CAD build for the part. Positions are in the model's coordinates, mm. A direction names the side the tool comes from. Give positions to 0.01 mm unless a question says otherwise; leave off trailing zeros. Loops run counter-clockwise (first coordinate to the right, second up) from the corner with the lowest first, then second, coordinate; pieces in that order, holes last.
```python
from build123d import *

# Parameters (mm, degrees)
BOSS_EXTRUDE1_DEPTH = 5.35
SKETCH2_R           = 5
BOSS_EXTRUDE2_DEPTH = 1
SKETCH3_R           = 3.555
BOSS_EXTRUDE3_DEPTH = 2.5
SKETCH4_R           = 2.5
CUT_EXTRUDE1_DEPTH  = 9.85
CUT_EXTRUDE2_DEPTH  = 4.5


with BuildPart() as part:
    # Sketch1 → Boss-Extrude1 (new body)
    with BuildSketch(Plane(origin=(0, 0, 0), x_dir=(1, 0, 0), z_dir=(0, 1, 0))):
        Polygon((4.543746619, 0), (2.271873309, 3.935), (-2.271873309, 3.935), (-4.543746619, 0), (-2.271873309, -3.935), (2.271873309, -3.935), align=None)
    extrude(amount=BOSS_EXTRUDE1_DEPTH)

    # Sketch2 → Boss-Extrude2 (add)
    with BuildSketch(Plane(origin=(0, 0, 0), x_dir=(1, 0, 0), z_dir=(0, 1, 0))):
        Circle(SKETCH2_R)
    extrude(amount=-BOSS_EXTRUDE2_DEPTH)

    # Sketch3 → Boss-Extrude3 (add)
    with BuildSketch(Plane.XZ.offset(1)):
        Circle(SKETCH3_R)
    extrude(amount=BOSS_EXTRUDE3_DEPTH)

    # Sketch4 → Cut-Extrude1 (cut, through all)
    with BuildSketch(Plane(origin=(0, 5.35, 0), x_dir=(1, 0, 0), z_dir=(0, 1, 0))):
        with Locations((0, -0.79)):
            Circle(SKETCH4_R)
    extrude(amount=-CUT_EXTRUDE1_DEPTH, mode=Mode.SUBTRACT)

    # Sketch5 → Cut-Extrude2 (cut, through all)
    with BuildSketch(Plane(origin=(0, 0, 0), x_dir=(1, 0, 0), z_dir=(0, 1, 0))):
        with BuildLine():
            Line((-1.7, -4.702127178), (0, -4.202127178))
            Line((0, -4.202127178), (1.7, -4.702127178))
            ThreePointArc((1.7, -4.702127178), (0, -5), (-1.7, -4.702127178))
        make_face()
    extrude(amount=-CUT_EXTRUDE2_DEPTH, mode=Mode.SUBTRACT)

    # Sketch6 → Cut-Revolve1 (revolve, cut)
    with BuildSketch(Plane.XY):
        Polygon((4.043746619, 5.35), (4.543746619, 5.35), (4.543746619, 4.85), align=None)
    revolve(axis=Axis((0, 0, 0), (0, 1, 0)), mode=Mode.SUBTRACT)


solid = part.part
```
1. Pull direction X, two halves, no side cores. Call faces 1 (the face through (-0.54, 0.99, 3.23)), 2 (the face through (0, 0, -4.1)), 3 (the face through (-2.075, 5.215, -3.628)), 4 (the face through (-0.862, -0.493, 4.456)): released by +X, released by -X, zero draft, split by the parting line, or undercut.
Responses:
face 1: undercut
face 2: zero draft
face 3: released by -X
face 4: undercut
2. Saw through at A-A, the plane y = 1.25. List the corners of the cut face in (x, z) (3 decimals), and give its area (3 significant figures).
Responses:
outline: (-4.544, 0) - (-2.272, -3.935) - (2.272, -3.935) - (4.544, 0) - (2.272, 3.935) - (-2.272, 3.935) - close; hole circle Ø5 at (0, 0.79)
area: 34.0 mm2
3. Drop flat-ended pins along their axis: pin 1 (2.5 mm diameter, centred on x = -0.5, y = 4, fed in from -Z) (3 decimals); pin 2 (1.5 mm diameter, centred on y = -1.5, z = 1.5, fed in from -X); pin 3 (1.5 mm diameter, centred on y = 2, z = -3, fed in from -X). Give the stop position or say it passes through.
Responses:
pin 1: stops at z = -3.935
pin 2: stops at x = -4.91
pin 3: stops at x = -3.24
4. Probe line 1 along Z through (x, y) = (0, 3.75) (3 decimals); line 2 along Y through (x, z) = (-3.25, -3.25); line 3 along Z through (x, y) = (0.5, -0.5). List the from-to ranges inside material, lowest first.
Responses:
line 1: z = -3.935 to -1.71, 3.29 to 3.935
line 2: y = -1 to 0
line 3: z = -4.97 to -1.66, 3.24 to 4.35
5. Tool access for faces 5 (the face through (0.84, -0.49, 4.45)), 6 (the face through (-3.424, 2.638, 1.94)), 7 (the face through (3.39, -2.23, 1.07)), 8 (the face through (0, 3, 3.935)): list every direction of +Z, -Z, +X, -X, +Y, -Y with a clear straight run to the whole face (end or side of a thin tool).
Responses:
face 5: +Z, +Y, -Y
face 6: +Z, -X, +Y
face 7: -Y
face 8: +Z, +X, -X, +Y
6. Saw through at C-C, the plane z = -2. List the corners of the cut face in (x, y).
Responses:
outline: (-4.58, -1) - (-2.94, -1) - (-2.94, -3.5) - (2.94, -3.5) - (2.94, -1) - (4.58, -1) - (4.58, 0) - (3.39, 0) - (3.39, 5.35) - (-3.39, 5.35) - (-3.39, 0) - (-4.58, 0) - close
7. Saw through at B-B, the plane z = 2.25. List the corners of the cut face in (x, y).
Responses:
outline: (-4.47, -1) - (-2.75, -1) - (-2.75, -3.5) - (-2.03, -3.5) - (-2.03, 5.35) - (-3.24, 5.35) - (-3.24, 0) - (-4.47, 0) - close; (2.03, -3.5) - (2.75, -3.5) - (2.75, -1) - (4.47, -1) - (4.47, 0) - (3.24, 0) - (3.24, 5.35) - (2.03, 5.35) - close
